```python
from build123d import *

# Parameters (mm, degrees)
SKETCH6_W                    = 50
SKETCH6_H                    = 40
BASE_FLANGE2_DEPTH           = 1.4
CUT_EXTRUDE2_DEPTH           = 65.046545574
CUT_EXTRUDE2_DEPTH_BACK      = 65.046545574
SKETCH11_R                   = 7.5
SKETCH11_R_2                 = 1.7
EDGE_FLANGE1_STRIP_W         = 11.6
EDGE_FLANGE1_STRIP_H         = 1.4
EDGE_FLANGE1_STRIP_CUT_DEPTH = 50
EDGE_FLANGE1_DEPTH           = 50
SKETCH35_R                   = 2
CUT_EXTRUDE3_DEPTH           = 75.766035069


# Sheet-metal steps are written as plain solids
with BuildPart() as part:
    # Sketch6 → Base-Flange2 (new body)
    with BuildSketch(Plane.XY):
        with Locations((25, 20)):
            Rectangle(SKETCH6_W, SKETCH6_H)
    extrude(amount=-BASE_FLANGE2_DEPTH)

    # Sketch11 → Cut-Extrude2 (cut, two sides: drawn at the far end of the back side and taken through both)
    with BuildSketch(Plane.XY.offset(-1.4).offset(-CUT_EXTRUDE2_DEPTH_BACK)):
        with Locations((25, 20)):
            Circle(SKETCH11_R)
        with Locations((25, 30)):
            Circle(SKETCH11_R_2)
        with Locations((16.339745962, 15)):
            Circle(SKETCH11_R_2)
        with Locations((33.660254038, 15)):
            Circle(SKETCH11_R_2)
    extrude(amount=CUT_EXTRUDE2_DEPTH + CUT_EXTRUDE2_DEPTH_BACK, mode=Mode.SUBTRACT)

    # Edge-Flange1 strip (across the edge) → Edge-Flange1 strip cut (cut)
    with BuildSketch(Plane(origin=(50, 0, -1.4), x_dir=(0, 1, 0), z_dir=(-1, 0, 0))):
        with Locations((-1.4, -0.7)):
            Rectangle(EDGE_FLANGE1_STRIP_W, EDGE_FLANGE1_STRIP_H)
    extrude(amount=EDGE_FLANGE1_STRIP_CUT_DEPTH, mode=Mode.SUBTRACT)

    # Edge-Flange1 section (across the edge) → Edge-Flange1 (add)
    with BuildSketch(Plane(origin=(50, 0, -1.4), x_dir=(0, 1, 0), z_dir=(-1, 0, 0))):
        with BuildLine():
            Line((0, 3), (0, 38.6))
            Line((0, 38.6), (1.4, 38.6))
            Line((1.4, 38.6), (1.4, 3))
            ThreePointArc((1.4, 3), (2.278679656, 0.878679656), (4.4, 0))
            Line((4.4, 0), (4.4, -1.4))
            ThreePointArc((4.4, -1.4), (1.288730163, -0.111269837), (0, 3))
        make_face()
    extrude(amount=EDGE_FLANGE1_DEPTH)

    # Sketch35 → Cut-Extrude3 (cut, through all)
    with BuildSketch(Plane(origin=(0, 1.4, 0), x_dir=(1, 0, 0), z_dir=(0, 1, 0))):
        with Locations(Location((43, 11.4, 0), (0, 0, 270))):
            Circle(SKETCH35_R)
        with Locations(Location((7, 11.4, 0), (0, 0, 270))):
            Circle(SKETCH35_R)
        with Locations(Location((43, 33, 0), (0, 0, 270))):
            Circle(SKETCH35_R)
        with Locations(Location((7, 33, 0), (0, 0, 270))):
            Circle(SKETCH35_R)
    extrude(amount=-CUT_EXTRUDE3_DEPTH, mode=Mode.SUBTRACT)


solid = part.part
```
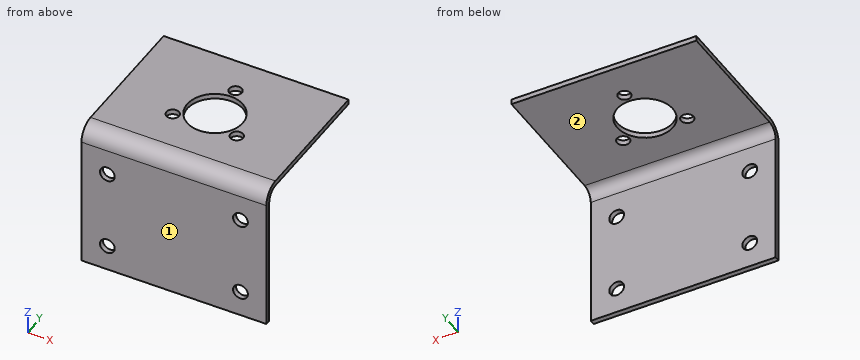
Geometry check sheet. Reference: the model listing, model coordinates, mm. Face numbers are marked on the shaded views. A direction names the side the tool comes from. Coordinates: 2 decimals unless noted, no trailing zeros. Write each loop counter-clockwise with the first axis right and the second up, starting at its lowest first coordinate (ties: lowest second). Pieces come first, ordered by that corner, then holes. Notation, with made-up numbers: M 64,15.5 L 116,15.5 A25 cw 116,30.5 Z; hole C 37,-16 d8. An arc over 180 degrees is marked long. Use one line per item in the form item = value. Start each with the question number.
1) Thickness scan on probe 1 along X at (y, z) = (0.3, -33); probe 2 along X at (y, z) = (15, -1); probe 3 along Y at (x, z) = (18, -18). Record the ranges inside material, lowest first. Write a range as from..to.
2) Section check C-C on z = -11.4. Enter the section's corners in (x, y), and give its area (3 significant figures).
3) Go/stop test with flat-tipped pins: pin 1 Ø1.5 at (x, y) = (9, 29) entering from -Z; pin 2 Ø6 at (x, y) = (21, 6) entering from -Z; pin 3 Ø1.5 at (x, z) = (15.5, -25.5) entering from +Y. Record where each tip stops, or that it passes through.
4) Section check D-D on x = 7. Enter the section's corners in (y, z), and give its area (3 significant figures).
5) Section check A-A on x = 25. Enter the section's corners in (y, z).
6) Section check B-B on y = 20. Enter the section's corners in (x, z).
7) Set-up check for the marked faces 1 and 2: record each of +Z, -Z, +X, -X, +Y, -Y from which the full face is reachable in a straight line by a thin tool's end or side.
Responses:
q1.probe_1 = 0..5, 9..41, 45..50
q1.probe_2 = 0..14.64, 18.04..19.41, 30.59..31.96, 35.36..50
q1.probe_3 = 0..1.4
q2.outline = M 0,0 L 5,0 L 5,1.4 L 0,1.4 Z; M 9,0 L 41,0 L 41,1.4 L 9,1.4 Z; M 45,0 L 50,0 L 50,1.4 L 45,1.4 Z
q2.area = 58.8 mm2
q3.pin_1 = -1.4
q3.pin_2 = -1.75
q3.pin_3 = 1.4
q4.outline = M 0,-40 L 1.4,-40 L 1.4,-35 L 0,-35 Z; M 0,-31 L 1.4,-31 L 1.4,-13.4 L 0,-13.4 Z; M 0,-9.4 L 1.4,-9.4 L 1.4,-4.4 A3 cw 4.4,-1.4 L 40,-1.4 L 40,0 L 4.4,0 A4.4 ccw 0,-4.4 Z
q4.area = 96.6 mm2
q5.outline = M 0,-40 L 1.4,-40 L 1.4,-4.4 A3 cw 4.4,-1.4 L 12.5,-1.4 L 12.5,0 L 4.4,0 A4.4 ccw 0,-4.4 Z; M 27.5,-1.4 L 28.3,-1.4 L 28.3,0 L 27.5,0 Z; M 31.7,-1.4 L 40,-1.4 L 40,0 L 31.7,0 Z
q6.outline = M 0,-1.4 L 17.5,-1.4 L 17.5,0 L 0,0 Z; M 32.5,-1.4 L 50,-1.4 L 50,0 L 32.5,0 Z
q7.face_1 = +Z, -Z, +X, -X, -Y
q7.face_2 = -Z, +X, -X, +Y
